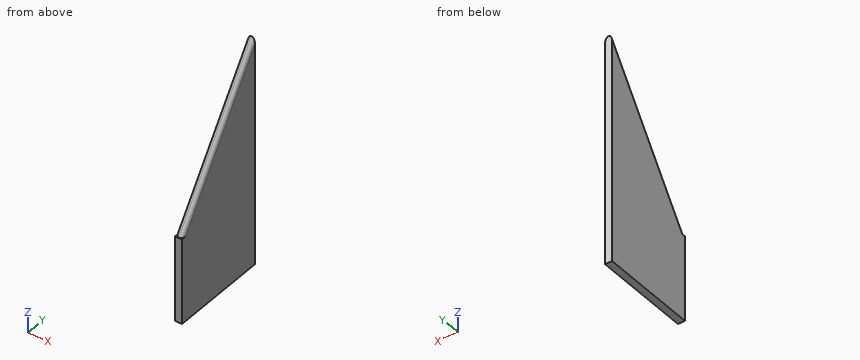
from build123d import *

# Parameters (mm, degrees)
F0_W     = 0.6239625519
F0_H     = 120
F1_DEPTH = 10
F2_R     = 4.99999


# Not quite as in the source:
# - a fillet or chamfer is up to 0.001 mm smaller than in the source, because OpenCascade refuses the exact size


with BuildPart() as f1:
    # F0 (on Right) → F1 (new body)
    with BuildSketch(Plane.YZ):
        with Locations((-139.943079155, 60)):
            Rectangle(F0_W, F0_H)
        Polygon((-139.631097879, 120), (-139.631097879, 0), (0, 0), (0, 321.3160612199), align=None)
    extrude(amount=F1_DEPTH)

    # F2 (radius 5 in the source; OpenCascade refuses exactly that, so slightly less here)
    f2_edges = [f1.edges().sort_by_distance(p)[0] for p in [
        (10, -69.815549, 220.658031),
        (0, -69.815549, 220.658031),
    ]]
    fillet(f2_edges, radius=F2_R)


solid = f1.part
For this review, take the finished solid that the model builds, in its own axes (mm). Round coordinates to 2 decimals unless told otherwise and drop trailing zeros. Order: outer loops, then holes, each group sorted by start corner. A loop starts at its lowest first (then second) coordinate and runs counter-clockwise, first axis right, second up. Notation, with made-up numbers: M 9.25,79.25 L 68.25,79.25 A10 ccw 68.25,93.25 Z; hole C 61.5,23 d7. An arc over 180 degrees is marked long. Use a Markdown table: item, result. Add a question column.
Item 1: To check wall thickness, follow line 1 along Z through (x, y) = (1.5, -39); line 2 along Z through (x, y) = (5.5, -42); line 3 along Y through (x, z) = (2, 277). State the ranges of each line that lie inside material, in increasing order.
Item 2: Add section A-A, the plane x = 8.5. Give the boundary of the cut face in (y, z).
Item 3: Insertion check: pin 1 (2 mm diameter, centred on x = 9, y = -22, fed in from +Z); pin 2 (3 mm diameter, centred on x = 1, z = 132.5, fed in from -Y); pin 3 (2 mm diameter, centred on x = 6.5, z = 281, fed in from -Y). Each pin has a flat end and moves straight along its axis. Give the tip position at first contact, or say it passes through.
Geometry results:
| question | item | result |
|---|---|---|
| 1 | line 1 | z = 0 to 262.58 |
| 1 | line 2 | z = 0 to 260.72 |
| 1 | line 3 | y = -29.52 to 0 |
| 2 | outline | M -140.26,0 L 0,0 L 0,318.81 L -137.89,120 L -140.26,120 Z |
| 3 | pin 1 | stops at z = 288.45 |
| 3 | pin 2 | stops at y = -130.54 |
| 3 | pin 3 | stops at y = -28.45 |
